For this review, take the finished solid that the model builds, in its own axes (mm). Give positions to 0.01 mm unless a question says otherwise; leave off trailing zeros. Loops run counter-clockwise (first coordinate to the right, second up) from the corner with the lowest first, then second, coordinate; pieces in that order, holes last. Notation, with made-up numbers: (-16.5, 76.25) - (-4.5, 76.25) arc R5 cw to (-4.5, 85.25) - close; hole circle Ø3 at (81.5, 81.25). An arc over 180 degrees is marked (long way). Answer in a Markdown table with one row per item.
```python
from build123d import *

# Parameters (mm, degrees)
SKETCH_1_W          = 58
SKETCH_1_H          = 100
SKETCH_1_R          = 1
SKETCH_1_R_2        = 1.5
EXTRUDE_1_DEPTH     = 2.5
SKETCH_2_R          = 1.5
SKETCH_2_R_2        = 19
CUT_EXTRUDE_1_DEPTH = 10
SKETCH_2_3_W        = 30
SKETCH_2_3_H        = 100
SKETCH_2_3_W_2      = 32
EXTRUDE_2_DEPTH     = 2.5
FILLET_1_R          = 30
FILLET_2_R          = 10
SKETCH_4_R          = 4
SKETCH_4_R_2        = 1
SKETCH_4_R_3        = 1.5
CUT_EXTRUDE_3_DEPTH = 10


with BuildPart() as part:
    # Sketch 1 → Extrude 1 (new body)
    with BuildSketch(Plane.XY):
        Rectangle(SKETCH_1_W, SKETCH_1_H)
        with Locations((-24, 48.25)):
            Circle(SKETCH_1_R, mode=Mode.SUBTRACT)
        with Locations((-16, 48.25)):
            Circle(SKETCH_1_R_2, mode=Mode.SUBTRACT)
        with Locations(Location((16, 48.25, 0), (0, 0, 180))):
            Circle(SKETCH_1_R_2, mode=Mode.SUBTRACT)
        with Locations(Location((24, 48.25, 0), (0, 0, 180))):
            Circle(SKETCH_1_R, mode=Mode.SUBTRACT)
        with Locations((-19.7, 28.75)):
            Circle(SKETCH_1_R, mode=Mode.SUBTRACT)
        with Locations((-25.7, 28.75)):
            Circle(SKETCH_1_R_2, mode=Mode.SUBTRACT)
        with Locations(Location((19.7, 28.75, 0), (0, 0, 180))):
            Circle(SKETCH_1_R, mode=Mode.SUBTRACT)
        with Locations(Location((25.7, 28.75, 0), (0, 0, 180))):
            Circle(SKETCH_1_R_2, mode=Mode.SUBTRACT)
        with Locations((25.7, -28.75)):
            Circle(SKETCH_1_R_2, mode=Mode.SUBTRACT)
        with Locations((24, -48.25)):
            Circle(SKETCH_1_R, mode=Mode.SUBTRACT)
        with Locations((16, -48.25)):
            Circle(SKETCH_1_R_2, mode=Mode.SUBTRACT)
        with Locations((19.7, -28.75)):
            Circle(SKETCH_1_R, mode=Mode.SUBTRACT)
        with Locations(Location((-19.7, -28.75, 0), (0, 0, 180))):
            Circle(SKETCH_1_R, mode=Mode.SUBTRACT)
        with Locations(Location((-25.7, -28.75, 0), (0, 0, 180))):
            Circle(SKETCH_1_R_2, mode=Mode.SUBTRACT)
        with Locations(Location((-24, -48.25, 0), (0, 0, 180))):
            Circle(SKETCH_1_R, mode=Mode.SUBTRACT)
        with Locations(Location((-16, -48.25, 0), (0, 0, 180))):
            Circle(SKETCH_1_R_2, mode=Mode.SUBTRACT)
    extrude(amount=EXTRUDE_1_DEPTH)

    # Sketch 2 → Cut-Extrude 1 (cut)
    with BuildSketch(Plane.XY.offset(2.5)):
        with Locations((0, -22)):
            Circle(SKETCH_2_R)
        with Locations((-22, 0)):
            Circle(SKETCH_2_R)
        with Locations((0, 22)):
            Circle(SKETCH_2_R)
        Circle(SKETCH_2_R_2)
        with Locations((22, 0)):
            Circle(SKETCH_2_R)
    extrude(amount=-CUT_EXTRUDE_1_DEPTH, mode=Mode.SUBTRACT)

    # Sketch 2_3 → Extrude 2 (add)
    with BuildSketch(Plane.XY.offset(2.5)):
        with Locations((-44, 0)):
            Rectangle(SKETCH_2_3_W, SKETCH_2_3_H)
        with Locations((45, 0)):
            Rectangle(SKETCH_2_3_W_2, SKETCH_2_3_H)
    extrude(amount=-EXTRUDE_2_DEPTH)

    # Fillet 1
    fillet_1_edges = [part.edges().sort_by_distance(p)[0] for p in [
        (-59, -50, 1.25),
        (-59, 50, 1.25),
    ]]
    fillet(fillet_1_edges, radius=FILLET_1_R)

    # Fillet 2
    fillet_2_edges = [part.edges().sort_by_distance(p)[0] for p in [
        (61, 50, 1.25),
        (61, -50, 1.25),
    ]]
    fillet(fillet_2_edges, radius=FILLET_2_R)

    # Sketch 4 → Cut-Extrude 3 (cut)
    with BuildSketch(Plane.XY.offset(2.5)):
        with Locations((55, 0)):
            Circle(SKETCH_4_R)
        with Locations((55, 10)):
            Circle(SKETCH_4_R_2)
        with Locations((55, -10)):
            Circle(SKETCH_4_R_2)
        with Locations((45, 0)):
            Circle(SKETCH_4_R_2)
        with Locations((-54, 5)):
            Circle(SKETCH_4_R_3)
        with Locations((-54, -5)):
            Circle(SKETCH_4_R_3)
        with Locations((-50.846052275, 35)):
            Circle(SKETCH_4_R_3)
        with Locations((56, -40)):
            Circle(SKETCH_4_R_3)
        with Locations((-50.846052275, -35)):
            Circle(SKETCH_4_R_3)
        with Locations((56, 40)):
            Circle(SKETCH_4_R_3)
        with Locations((-47, 0)):
            Circle(SKETCH_4_R_3)
        with BuildLine():
            Line((-42.5, -15), (-42.5, 15))
            ThreePointArc((-42.5, 15), (-41, 16.5), (-39.5, 15))
            Line((-39.5, 15), (-39.5, -15))
            ThreePointArc((-39.5, -15), (-41, -16.5), (-42.5, -15))
        make_face()
        with BuildLine():
            Line((-33, -15), (-33, 15))
            ThreePointArc((-33, 15), (-31.5, 16.5), (-30, 15))
            Line((-30, 15), (-30, -15))
            ThreePointArc((-30, -15), (-31.5, -16.5), (-33, -15))
        make_face()
        with BuildLine():
            Line((26.5, -15), (26.5, 15))
            ThreePointArc((26.5, 15), (28, 16.5), (29.5, 15))
            Line((29.5, 15), (29.5, -15))
            ThreePointArc((29.5, -15), (28, -16.5), (26.5, -15))
        make_face()
        with BuildLine():
            Line((34.5, -15), (34.5, 15))
            ThreePointArc((34.5, 15), (36, 16.5), (37.5, 15))
            Line((37.5, 15), (37.5, -15))
            ThreePointArc((37.5, -15), (36, -16.5), (34.5, -15))
        make_face()
    extrude(amount=-CUT_EXTRUDE_3_DEPTH, mode=Mode.SUBTRACT)


solid = part.part
```
1. We need section D-D, the plane x = -37.5. Give the boundary of the cut face in (y, z).
Values:
| item | result |
|---|---|
| outline | (-48.77, 0) - (48.77, 0) - (48.77, 2.5) - (-48.77, 2.5) - close |
2. We need section B-B, the plane y = -35. Give the boundary of the cut face in (x, z).
Values:
| item | result |
|---|---|
| outline | (-54.98, 0) - (-52.35, 0) - (-52.35, 2.5) - (-54.98, 2.5) - close; (-49.35, 0) - (61, 0) - (61, 2.5) - (-49.35, 2.5) - close |
3. We need section A-A, the plane x = 36. Give the boundary of the cut face in (y, z).
Values:
| item | result |
|---|---|
| outline | (-50, 0) - (-16.5, 0) - (-16.5, 2.5) - (-50, 2.5) - close; (16.5, 0) - (50, 0) - (50, 2.5) - (16.5, 2.5) - close |
4. Mouldability with a two-part tool opening along X and no side actions: class faces 1 (the face through (-59, 0, 1)), 2 (the face through (56.69, -41.33, 1.27)), 3 (the face through (13, -22, 2.5)) as released by +X, released by -X, zero draft, split by the parting line, or undercut.
Values:
| item | result |
|---|---|
| face 1 | released by -X |
| face 2 | undercut |
| face 3 | zero draft |
5. Wall thickness on line 1 (Y direction, x = 0, z = 1.35); line 2 (Y direction, x = -16, z = 1.5); line 3 (X direction, y = 28, z = 2.3): over which ranges is each line inside the solid? List them lowest first. Write a range as [from, to].
Values:
| item | result |
|---|---|
| line 1 | y = [-50, -23.5], [-20.5, -19], [19, 20.5], [23.5, 50] |
| line 2 | y = [-50, -49.75], [-46.75, -10.25], [10.25, 46.75], [49.75, 50] |
| line 3 | x = [-57.91, -27], [-24.4, -20.36], [-19.04, 19.04], [20.36, 24.4], [27, 61] |
6. We need section C-C, the plane z = 0.8. Count the separate pieces of the cut face and the enclosed holes in it, and give its area (3 significant figures).
Values:
| item | result |
|---|---|
| separate pieces | 1 |
| enclosed holes | 36 |
| area | 9,830 mm^2 |
7. Clearance check with a flat-ended pin moving along its axis: pin 1 (2.5 mm diameter, centred on x = 0, y = 22, fed in from +Z). State where the tip first meets the part, or that it passes through.
Values:
| item | result |
|---|---|
| pin 1 | passes through |
